The model under review builds one solid part; all positions refer to its coordinate system, in mm. A direction names the side the tool comes from. Coordinates: 2 decimals unless noted, no trailing zeros. Order: outer loops, then holes, each group sorted by start corner. A loop starts at its lowest first (then second) coordinate and runs counter-clockwise, first axis right, second up.
```python
from build123d import *

# Parameters (mm, degrees)
SKETCH2_W           = 19.7
SKETCH2_H           = 5
BOSS_EXTRUDE1_DEPTH = 5
BOSS_EXTRUDE2_DEPTH = 5
SKETCH5_R           = 0.85
CUT_EXTRUDE1_DEPTH  = 5


with BuildPart() as part:
    # Sketch2 → Boss-Extrude1 (new body)
    with BuildSketch(Plane(origin=(0, 0, 0), x_dir=(1, 0, 0), z_dir=(0, 1, 0))):
        with Locations((0, 2.5)):
            Rectangle(SKETCH2_W, SKETCH2_H)
    extrude(amount=BOSS_EXTRUDE1_DEPTH)

    # Sketch4 → Boss-Extrude2 (add)
    with BuildSketch(Plane.XY):
        Polygon((-16, 5), (16, 5), (16, 48), (0, 48), (-16, 48), align=None)
        Polygon((-12.5, 22.5), (12.5, 22.5), (12.5, 43), (0, 43), (-12.5, 43), align=None, mode=Mode.SUBTRACT)
    extrude(amount=-BOSS_EXTRUDE2_DEPTH)

    # Sketch5 → Cut-Extrude1 (cut)
    with BuildSketch(Plane.XY):
        with Locations((-14.05, 45.5)):
            Circle(SKETCH5_R)
        with Locations((-14.05, 17.4)):
            Circle(SKETCH5_R)
        with Locations((14.05, 17.4)):
            Circle(SKETCH5_R)
        with Locations((14.05, 45.5)):
            Circle(SKETCH5_R)
    extrude(amount=-CUT_EXTRUDE1_DEPTH, mode=Mode.SUBTRACT)


solid = part.part
```
(1) We need section B-B, the plane y = 29. Write out the cut boundary in (x, z), and give its area (3 significant figures).
A:
outline: (-16, -5) - (-12.5, -5) - (-12.5, 0) - (-16, 0) - close; (12.5, -5) - (16, -5) - (16, 0) - (12.5, 0) - close
area: 35.0 mm2
(2) We need section C-C, the plane z = -3.3. Write out the cut boundary in (x, y).
A:
outline: (-16, 5) - (-9.85, 5) - (-9.85, 0) - (9.85, 0) - (9.85, 5) - (16, 5) - (16, 48) - (-16, 48) - close; hole circle Ø1.7 at (-14.05, 17.4); hole circle Ø1.7 at (-14.05, 45.5); hole (-12.5, 22.5) - (12.5, 22.5) - (12.5, 43) - (-12.5, 43) - close; hole circle Ø1.7 at (14.05, 17.4); hole circle Ø1.7 at (14.05, 45.5)
(3) Draft analysis for pull direction X (two halves, no side actions). For faces 5 (the face through (-9.85, 2, -2)), 6 (the face through (0, 43, -2)), 7 (the face through (0, 0, -3)), state which applies: released by +X, released by -X, zero draft, split by the parting line, or undercut.
A:
face 5: released by -X
face 6: undercut
face 7: zero draft
(4) We need section D-D, the plane x = -6. Write out the cut boundary in (y, z).
A:
outline: (0, -5) - (22.5, -5) - (22.5, 0) - (0, 0) - close; (43, -5) - (48, -5) - (48, 0) - (43, 0) - close
(5) We need section A-A, the plane x = -14.05. Write out the cut boundary in (y, z), and give its area (3 significant figures).
A:
outline: (5, -5) - (16.55, -5) - (16.55, 0) - (5, 0) - close; (18.25, -5) - (44.65, -5) - (44.65, 0) - (18.25, 0) - close; (46.35, -5) - (48, -5) - (48, 0) - (46.35, 0) - close
area: 198 mm2
(6) Machinability: for faces 1 (the face through (12.5, 33, -2)), 2 (the face through (-13, 5, -2)), 3 (the face through (0, 19, -5)), 4 (the face through (13, 5, -2)), which of the approach directions +Z, -Z, +X, -X, +Y, -Y give a long, thin tool a straight path to every point of the face, cutting with its end or side? Answer none if there is none.
A:
face 1: +Z, -Z
face 2: +Z, -Z, -X, -Y
face 3: -Z, +X, -X, +Y, -Y
face 4: +Z, -Z, +X, -Y
(7) Wall thickness on probe 1 along X at (y, z) = (45.5, -3.4); probe 2 along Y at (x, z) = (14.05, -1.05); probe 3 along Y at (x, z) = (1.5, -0.6): over which ranges is each line inside the solid? List them lowest first.
A:
probe 1: x = -16 to -14.9, -13.2 to 13.2, 14.9 to 16
probe 2: y = 5 to 16.55, 18.25 to 44.65, 46.35 to 48
probe 3: y = 0 to 22.5, 43 to 48
(8) For pin 1 Ø2.5 at (x, z) = (0, -1.5) entering from -Y; pin 2 Ø1.5 at (y, z) = (2, -2) entering from -X; pin 3 Ø1.5 at (x, z) = (14, -2) entering from -Y, all flat-tipped, find the tip position at first contact; note any pin that passes through.
A:
pin 1: stops at y = 0
pin 2: stops at x = -9.85
pin 3: stops at y = 5
